Could you check a few things on this drawing? It's one solid part, dimensions in mm from its lowest x, y, z. A direction names the side the tool comes from. Round coordinates to 2 decimals unless told otherwise and drop trailing zeros. Write each loop counter-clockwise with the first axis right and the second up, starting at its lowest first coordinate (ties: lowest second). Pieces come first, ordered by that corner, then holes. Notation, with made-up numbers: (81.25, 84.5) -> (139.25, 84.5) arc R32 ccw to (139.25, 116.5) -> close; hole circle Ø5 at (73.5, 25). An arc over 180 degrees is marked (long way). Return JSON: item names as keys, results as strings.
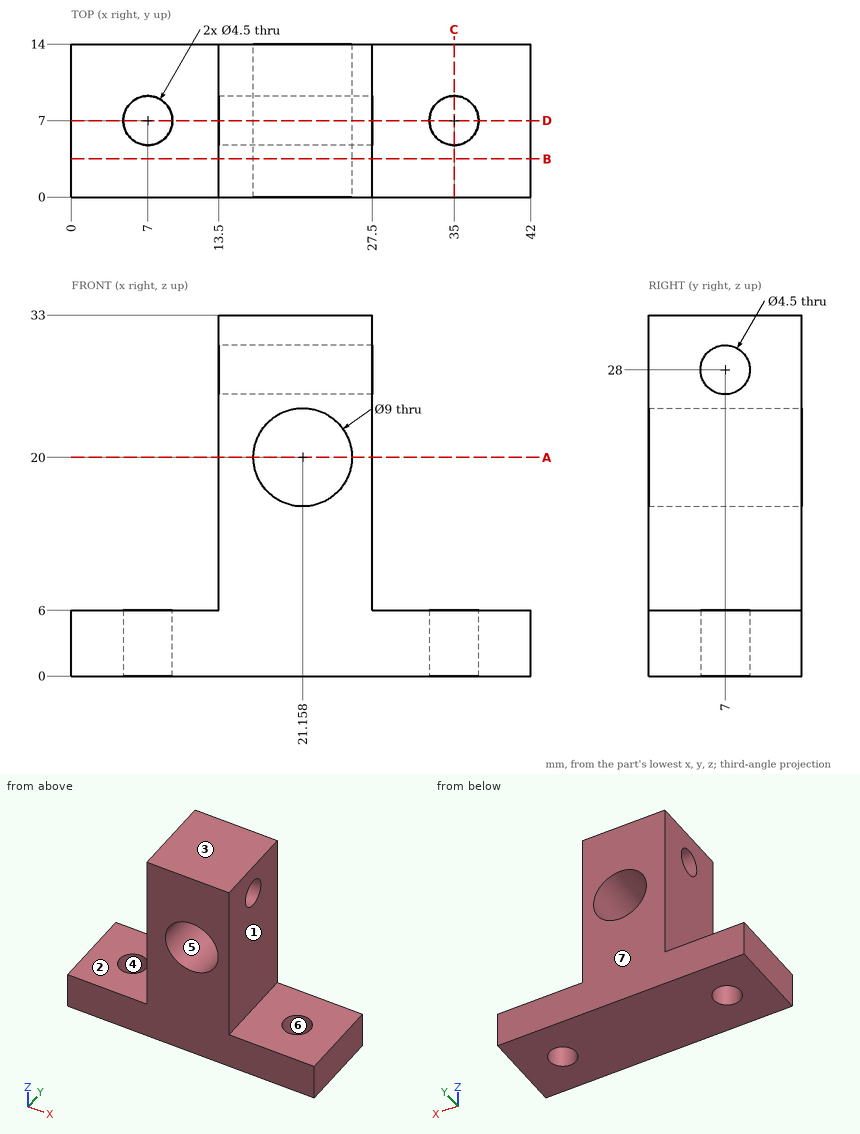
1) If I drill on probe 1 along X at (y, z) = (5.75, 20); probe 2 along Y at (x, z) = (35, 3.35); probe 3 along Z at (x, y) = (24, 9.5), over which ranges is the centre line in solid material (lowest first)? Write a range as [from, to].
Return value:
{"probe 1": "[13.5, 16.66], [25.66, 27.5]", "probe 2": "[0, 4.75], [9.25, 14]", "probe 3": "[0, 16.51], [23.49, 33]"}
2) Will these pins go through, and if not, where does the flat tip stop? pin 1 Ø4 at (y, z) = (7, 28) entering from +X; pin 2 Ø5 at (x, y) = (7, 7) entering from +Z; pin 3 Ø3 at (y, z) = (2, 10) entering from +X.
Return value:
{"pin 1": "through", "pin 2": "z = 6", "pin 3": "x = 27.5"}
3) I want a section at C-C, the plane x = 35. Please give me the cut outline in (y, z), and give its area (3 significant figures).
Return value:
{"outline": "(0, 0) -> (4.75, 0) -> (4.75, 6) -> (0, 6) -> close; (9.25, 0) -> (14, 0) -> (14, 6) -> (9.25, 6) -> close", "area": "57.0 mm²"}
4) I want a section at B-B, the plane y = 3.5. Please give me the cut outline in (x, z).
Return value:
{"outline": "(0, 0) -> (42, 0) -> (42, 6) -> (27.5, 6) -> (27.5, 33) -> (13.5, 33) -> (13.5, 6) -> (0, 6) -> close; hole circle Ø9 at (21.16, 20)"}
5) Thinking about a two-plate mould opening in Y: for the marked faces 4, 5, 6 and 7, which applies, pulls with the +Y half, pulls with the -Y half, needs draft (parallel to the pull), parting line crosses it, or undercut?
Return value:
{"face 4": "undercut", "face 5": "needs draft", "face 6": "undercut", "face 7": "pulls with the +Y half"}
6) I want a section at D-D, the plane y = 7. Please give me the cut outline in (x, z), and give its area (3 significant figures).
Return value:
{"outline": "(0, 0) -> (4.75, 0) -> (4.75, 6) -> (0, 6) -> close; (9.25, 0) -> (32.75, 0) -> (32.75, 6) -> (27.5, 6) -> (27.5, 25.75) -> (13.5, 25.75) -> (13.5, 6) -> (9.25, 6) -> close; (13.5, 30.25) -> (27.5, 30.25) -> (27.5, 33) -> (13.5, 33) -> close; (37.25, 0) -> (42, 0) -> (42, 6) -> (37.25, 6) -> close; hole circle Ø9 at (21.16, 20)", "area": "449 mm²"}
7) For the marked faces 1, 2 and 3, which set-ups out of +Z, -Z, +X, -X, +Y, -Y let a thin tool reach every point of the face, with its end or its side?
Return value:
{"face 1": "+Z, +X, +Y, -Y", "face 2": "+Z, -X, +Y, -Y", "face 3": "+Z, +X, -X, +Y, -Y"}
8) I want a section at A-A, the plane z = 20. Please give me the cut outline in (x, y), and give its area (3 significant figures).
Return value:
{"outline": "(13.5, 0) -> (16.66, 0) -> (16.66, 14) -> (13.5, 14) -> close; (25.66, 0) -> (27.5, 0) -> (27.5, 14) -> (25.66, 14) -> close", "area": "70.0 mm²"}
